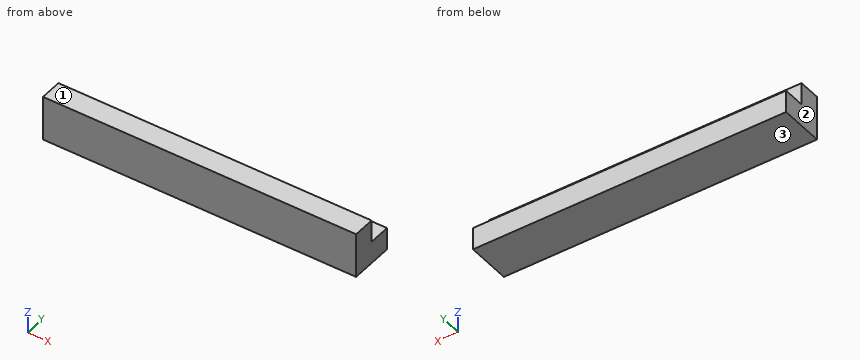
Autodesk Inventor part; units mm, degrees
ref_plane "YZ Plane" through (0, 0, 0) normal (1, 0, 0) x (0, 1, 0)
ref_plane "XZ Plane" through (0, 0, 0) normal (0, 1, 0) x (-1, 0, 0)
ref_plane "XY Plane" through (0, 0, 0) normal (0, 0, 1) x (1, 0, 0)
sketch "스케치1" plane through (0, 0, 0) normal (0, 0, 1) x (1, 0, 0)
  circle A0 centre (14.75, -25.8408) radius 14.2
  line L0 (41.95, 5.9) -> (41.95, -57.9408)
  line L1 (-41.95, 5.9) -> (41.95, 5.9)
  line L2 (-41.95, -57.9408) -> (-41.95, 5.9)
  line L3 (41.95, -57.9408) -> (-41.95, -57.9408)
  line L4 (-41.95, 5.9) -> (0, 5.9)
  line L5 (0, 5.9) -> (0, 0)
  line L6 (0, 0) -> (-41.95, 0)
  line L7 (-41.95, 0) -> (-41.95, 5.9)
  line L8 (-41.95, 0) -> (0, 0)
  line L9 (0, 0) -> (0, 2.95)
  line L10 (0, 2.95) -> (-41.95, 2.95)
  line L11 (-41.95, 2.95) -> (-41.95, 0)
extrude "돌출1" add sketch "스케치1" along normal blind 6 contours L5 L6 L2 L10
sketch "스케치2" plane through (-41.95, 0, 0) normal (-1, 0, 0) x (0, 0, 1)
  point P0 (0, 0)
sketch "스케치3" plane through (0, 0, 0) normal (0, 0, 1) x (1, 0, 0)
  point P0 (0, 0)
sketch "스케치4" plane through (0, 0, 0) normal (0, 0, 1) x (1, 0, 0)
  circle A0 centre (14.75, -25.8408) radius 14.2
  line L0 (41.95, 5.9) -> (41.95, -57.9408)
  line L1 (-41.95, 5.9) -> (41.95, 5.9)
  line L2 (-41.95, -57.9408) -> (-41.95, 5.9)
  line L3 (41.95, -57.9408) -> (-41.95, -57.9408)
  line L4 (-41.95, 5.9) -> (0, 5.9)
  line L5 (0, 5.9) -> (0, 2.95)
  line L6 (0, 2.95) -> (-41.95, 2.95)
  line L7 (-41.95, 2.95) -> (-41.95, 5.9)
  point P0 (0, 0)
  point P1 (0, 5.9)
extrude "돌출2" add sketch "스케치4" along normal blind 3 contours L5 L6 L2 L1
properties part number "부품73"
Source: CAD feature listing. Evaluate the final solid. Frame: model axes, mm. Face numbers are marked on the shaded views. Give positions to 0.01 mm unless a question says otherwise; leave off trailing zeros. Write each loop counter-clockwise with the first axis right and the second up, starting at its lowest first coordinate (ties: lowest second). Pieces come first, ordered by that corner, then holes.
1. First-contact query: pin 1 (3.5 mm diameter, centred on x = -25.5, z = 4.5, fed in from +Y); pin 2 (1.5 mm diameter, centred on x = -23, y = 4.5, fed in from +Z). Flat tips, straight axial feed; report the tip coordinate or a pass-through.
2. Section query A-A (z = 4.3). Return the cut outline in (x, y), then the cut area to 3 significant figures.
3. Section query B-B (x = -21). Return the cut outline in (y, z).
4. Pull-direction query (Z, two-part tool) for the marked faces 1, 2 and 3; classes: +Z half, -Z half, draft (parallel to the pull), parting line (faces both ways), or undercut.
5. Section query C-C (y = 4.2). Return the cut outline in (x, z).
6. Material intervals for line 1 along Z through (x, y) = (-22.5, 4.6); line 2 along Y through (x, z) = (-33.5, 3.95), sorted ascending.
Output values:
1. pin 1: stops at y = 5.9
1. pin 2: stops at z = 3
2. outline: (-41.95, 0) - (0, 0) - (0, 2.95) - (-41.95, 2.95) - close
2. area: 124 mm2
3. outline: (0, 0) - (5.9, 0) - (5.9, 3) - (2.95, 3) - (2.95, 6) - (0, 6) - close
4. face 1: +Z half
4. face 2: draft
4. face 3: -Z half
5. outline: (-41.95, 0) - (0, 0) - (0, 3) - (-41.95, 3) - close
6. line 1: z = 0 to 3
6. line 2: y = 0 to 2.95
